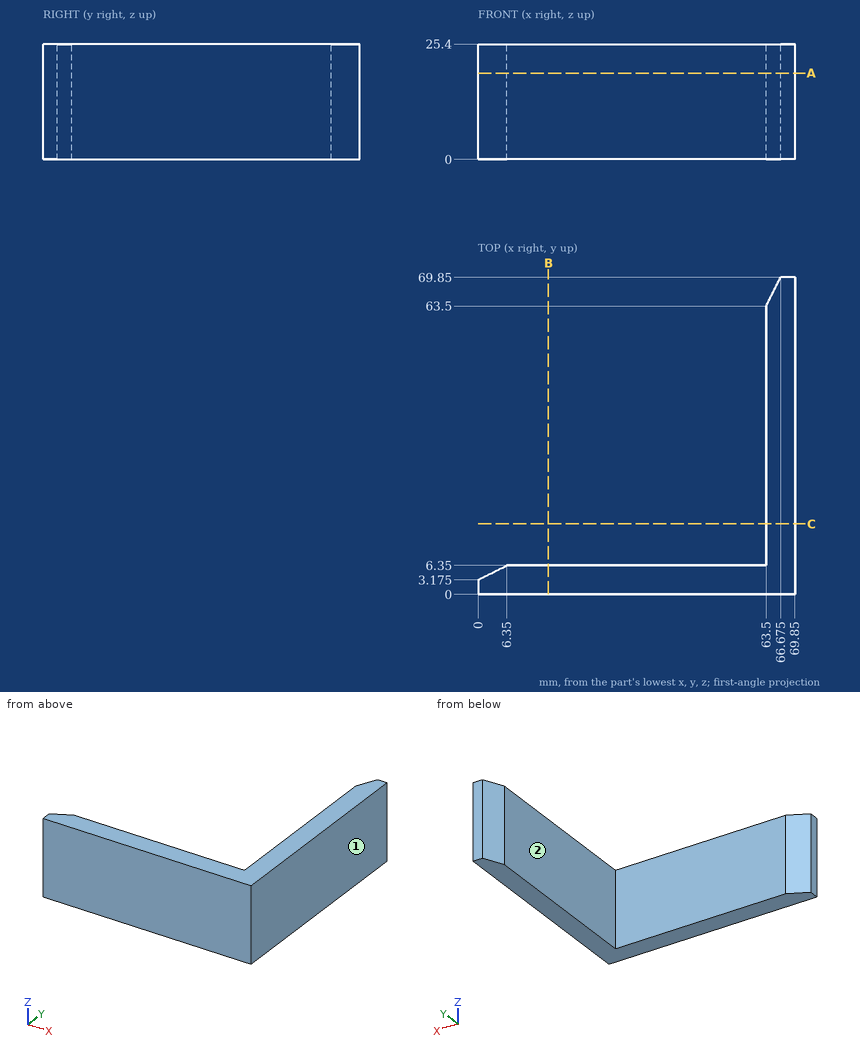
Source: three-view drawing plus pictorial views. Frame: mm from the lowest corner of the part. A direction names the side the tool comes from. Round coordinates to 2 decimals unless told otherwise and drop trailing zeros. Loops run counter-clockwise (first coordinate to the right, second up) from the corner with the lowest first, then second, coordinate; pieces in that order, holes last.
1. Section query A-A on z = 19. Output: boundary loops of the cut face in (x, y) (3 decimals), and give its area (3 significant figures).
2. Section query B-B on x = 15.5. Output: boundary loops of the cut face in (y, z).
3. Access query for the marked faces 1 and 2. Directions: +Z, -Z, +X, -X, +Y, -Y. A direction counts if a zero-diameter tool reaches every point of the face in a straight line with its end or side. Return the directions, or none.
4. Ray query, L1, parallel to Y at x = 37.5, z = 11.75; L2, parallel to X at y = 39, z = 14.5. Return the intervals inside material, ascending.
5. Section query C-C on y = 15.5. Output: boundary loops of the cut face in (x, z).
6. Contact query for a flat-ended pin moving along its axis: pin 1 (10 mm diameter, centred on x = 25.5, z = 13.5, fed in from +Y). Output: stop coordinate, or through.
Answers below:
1. outline: (0, 0) - (69.85, 0) - (69.85, 69.85) - (66.675, 69.85) - (63.5, 63.5) - (63.5, 6.35) - (6.35, 6.35) - (0, 3.175) - close
1. area: 827 mm2
2. outline: (0, 0) - (6.35, 0) - (6.35, 25.4) - (0, 25.4) - close
3. face 1: +Z, -Z, +X, +Y, -Y
3. face 2: +Z, -Z, -X, +Y
4. L1: y = 0 to 6.35
4. L2: x = 63.5 to 69.85
5. outline: (63.5, 0) - (69.85, 0) - (69.85, 25.4) - (63.5, 25.4) - close
6. pin 1: stops at y = 6.35
